Geometry: final body of the model. Coordinates: model frame, mm. Give positions to 0.01 mm unless a question says otherwise; leave off trailing zeros. Loops run counter-clockwise (first coordinate to the right, second up) from the corner with the lowest first, then second, coordinate; pieces in that order, holes last.
from build123d import *

# Parameters (mm, degrees)
ESQUISSE1_W             = 165
ESQUISSE1_H             = 6
BOSS_EXTRU_1_DEPTH      = 6
ESQUISSE2_R             = 1.5
ESQUISSE2_R_2           = 1
ENL_V_MAT_EXTRU_1_DEPTH = 166.218037756
CONG_1_R                = 2


with BuildPart() as part:
    # Esquisse1 → Boss.-Extru.1 (new body)
    with BuildSketch(Plane.XY):
        with Locations((82.5, 3)):
            Rectangle(ESQUISSE1_W, ESQUISSE1_H)
    extrude(amount=BOSS_EXTRU_1_DEPTH)

    # Esquisse2 → Enlèv. mat.-Extru.1 (cut, through all)
    with BuildSketch(Plane.XY.offset(6)):
        with Locations((162, 3)):
            Circle(ESQUISSE2_R)
        with Locations((2, 3)):
            Circle(ESQUISSE2_R_2)
    extrude(amount=-ENL_V_MAT_EXTRU_1_DEPTH, mode=Mode.SUBTRACT)

    # Congé1
    cong_1_edges = [part.edges().sort_by_distance(p)[0] for p in [
        (0, 6, 3),
        (165, 6, 3),
        (165, 0, 3),
        (0, 0, 3),
    ]]
    fillet(cong_1_edges, radius=CONG_1_R)


solid = part.part
Item 1: Pin query (flat end, axial travel): pin 1 (1.2 mm diameter, centred on x = 2, y = 3, fed in from +Z); pin 2 (1 mm diameter, centred on y = 5, z = 4.5, fed in from -X). Return the tip coordinate at first contact, or that it passes through.
Values follow:
pin 1: passes through
pin 2: stops at x = 0.06
Item 2: Ray query, probe 1 along X at (y, z) = (3.05, 2.5); probe 2 along Y at (x, z) = (2, 1.55); probe 3 along X at (y, z) = (2.15, 3.75). Return the intervals inside material, ascending.
Values follow:
probe 1: x = 0 to 1, 3 to 160.5, 163.5 to 165
probe 2: y = 0 to 2, 4 to 6
probe 3: x = 0 to 1.47, 2.53 to 160.76, 163.24 to 165
Item 3: Draft query along X for faces 1 (the face through (81, 3, 6)), 2 (the face through (163.386, 2.425, 3.042)). Return one class per face: +X half, -X half, draft (parallel to the pull), parting line (faces both ways), or undercut.
Values follow:
face 1: draft
face 2: undercut
Item 4: Section query A-A on y = 3. Return loops of the section in (x, z).
Values follow:
outline: (0, 0) - (1, 0) - (1, 6) - (0, 6) - close; (3, 0) - (160.5, 0) - (160.5, 6) - (3, 6) - close; (163.5, 0) - (165, 0) - (165, 6) - (163.5, 6) - close
